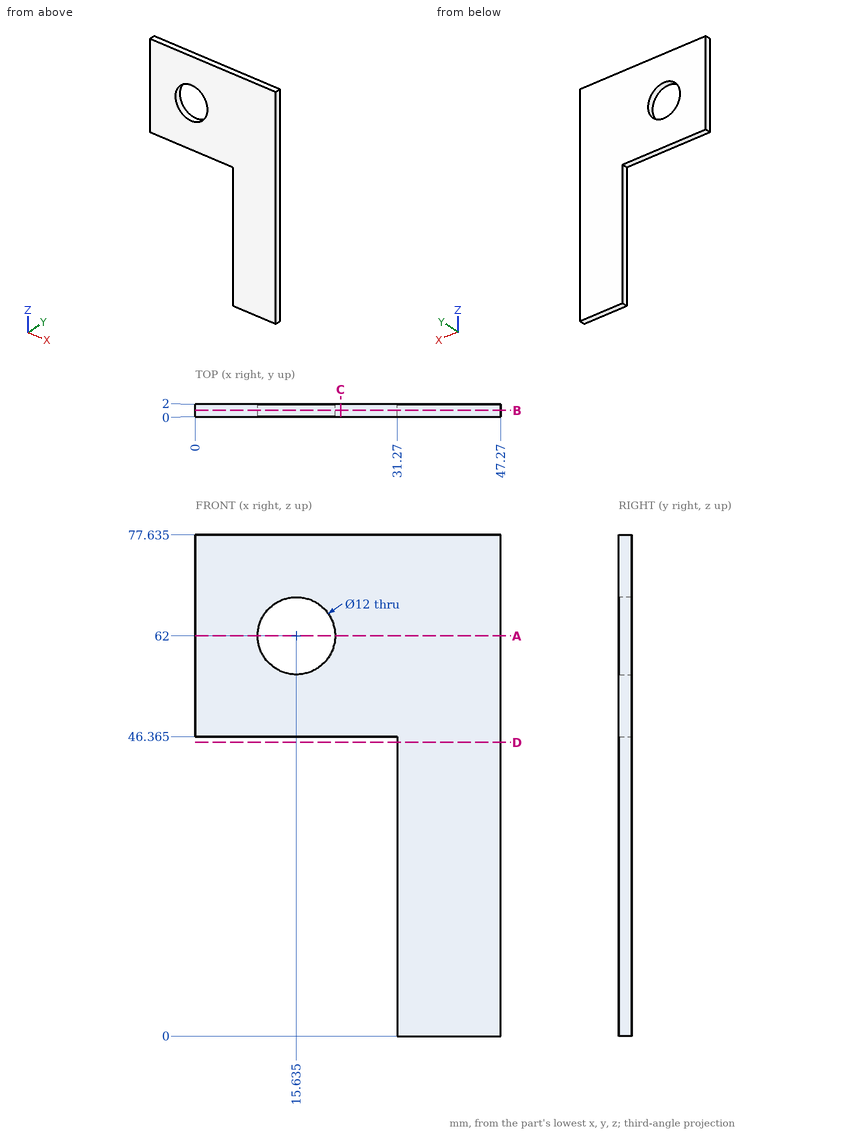
Answer from the drawing. Dimensions are ordinates in mm from the lowest x, y and z of the part. Coordinates: 2 decimals unless noted, no trailing zeros. Order: outer loops, then holes, each group sorted by start corner. A loop starts at its lowest first (then second) coordinate and runs counter-clockwise, first axis right, second up. Notation, with made-up numbers: M 39.25,10 L 47.25,10 A16 cw 47.25,37 Z; hole C 77.5,1 d5. An arc over 180 degrees is marked long. Put each result on its own line as item: value. Start each with the question number.
Item 1: Section B-B, the plane y = 1 is taken. Determine the outline of the cut face in (x, z) (3 decimals).
Item 2: Section A-A, the plane z = 62 is taken. Determine the outline of the cut face in (x, y) (3 decimals), plus the area to 3 significant figures.
Item 3: Section C-C, the plane x = 22.5 is taken. Determine the outline of the cut face in (y, z) (3 decimals), plus the area to 3 significant figures.
Item 4: Given pin 1 Ø12 at (x, z) = (11, 49.5) entering from -Y; pin 2 Ø1 at (y, z) = (0.5, 15) entering from -X; pin 3 Ø11 at (x, z) = (15.635, 62) entering from -Y, each flat-ended and moving along its own axis, determine where each tip first touches the part or whether it passes through.
Item 5: Consider probe 1 along X at (y, z) = (1.15, 62) (3 decimals); probe 2 along Z at (x, y) = (31, 1.45) (3 decimals); probe 3 along X at (y, z) = (0.6, 26). Determine where each line is inside the solid, lowest interval first. Write a range as [from, to].
Item 6: Section D-D, the plane z = 45.5 is taken. Determine the outline of the cut face in (x, y), plus the area to 3 significant figures.
Computed:
1. outline: M 0,46.365 L 31.27,46.365 L 31.27,0 L 47.27,0 L 47.27,77.635 L 0,77.635 Z; hole C 15.635,62 d12
2. outline: M 0,0 L 9.635,0 L 9.635,2 L 0,2 Z; M 21.635,0 L 47.27,0 L 47.27,2 L 21.635,2 Z
2. area: 70.5 mm2
3. outline: M 0,46.365 L 2,46.365 L 2,77.635 L 0,77.635 Z
3. area: 62.5 mm2
4. pin 1: stops at y = 0
4. pin 2: stops at x = 31.27
4. pin 3: passes through
5. probe 1: x = [0, 9.635], [21.635, 47.27]
5. probe 2: z = [46.365, 77.635]
5. probe 3: x = [31.27, 47.27]
6. outline: M 31.27,0 L 47.27,0 L 47.27,2 L 31.27,2 Z
6. area: 32.0 mm2
